The listing builds one solid part. Answer for the finished solid, in the listing's coordinates (mm). Coordinates: 2 decimals unless noted, no trailing zeros. Write each loop counter-clockwise with the first axis right and the second up, starting at its lowest first coordinate (ties: lowest second). Pieces come first, ordered by that corner, then holes. Notation, with made-up numbers: M 57.5,15 L 66.5,15 A17 ccw 66.5,32 Z; hole C -1,-38 d6. An arc over 180 degrees is marked long. Answer as CSV lines item,"result".
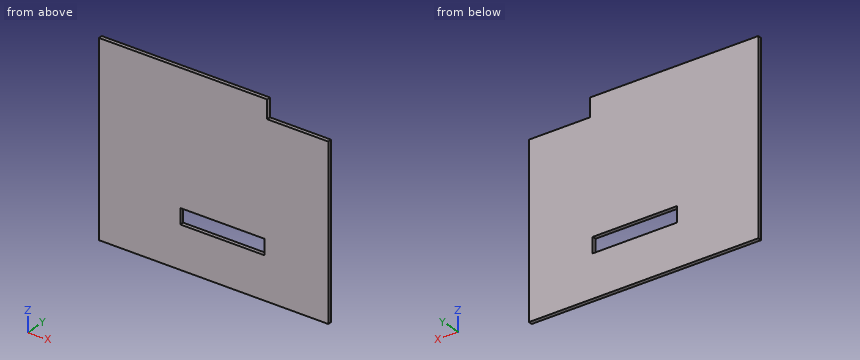
Autodesk Inventor part; units mm, degrees
ref_plane "YZ Plane" through (0, 0, 0) normal (1, 0, 0) x (0, 1, 0)
ref_plane "XZ Plane" through (0, 0, 0) normal (0, 1, 0) x (-1, 0, 0)
ref_plane "XY Plane" through (0, 0, 0) normal (0, 0, 1) x (1, 0, 0)
sketch "Esquisse1" plane through (0, 0, 0) normal (0, 1, 0) x (-1, 0, 0)
  line L0 (100.2268, 60.494) -> (-119.7732, 60.494)
  line L1 (-199.7732, 36.494) -> (-199.7732, -184.506)
  line L2 (-199.7732, -184.506) -> (100.2268, -184.506)
  line L3 (100.2268, -184.506) -> (100.2268, 60.494)
  line L4 (-119.7732, 60.494) -> (-119.7732, 36.494)
  line L5 (-119.7732, 36.494) -> (-199.7732, 36.494)
  point P0 (0, 0)
  dimension "d0" = 245
  dimension "d1" = 300
  dimension "d4" = 221
  dimension "d5" = 80
extrude "Extrusion1" add sketch "Esquisse1" along normal blind 5
sketch "Esquisse2" plane through (0, 5, 0) normal (0, 1, 0) x (1, 0, 0)
  line L0 (6.299, 109.506) -> (116.299, 109.506)
  line L1 (116.299, 109.506) -> (116.299, 129.506)
  line L2 (116.299, 129.506) -> (6.299, 129.506)
  line L3 (6.299, 129.506) -> (6.299, 109.506)
  line L4 (199.7732, 184.506) -> (-100.2268, 184.506)
  point P0 (0, 0)
  dimension "d6" = 20
  dimension "d7" = 110
  dimension "d8" = 55
extrude "Extrusion2" cut sketch "Esquisse2" against normal through all
properties part number "cote"
Q1. Find section C-C (y = 3.65). Give the vertices of the cut face in (x, z), and give its area (3 significant figures).
Output:
outline,"M -100.23,-184.51 L 199.77,-184.51 L 199.77,36.49 L 119.77,36.49 L 119.77,60.49 L -100.23,60.49 Z; hole M 6.3,-129.51 L 116.3,-129.51 L 116.3,-109.51 L 6.3,-109.51 Z"
area,"69,400 mm2"
Q2. Find section A-A (z = -116). Give the vertices of the cut face in (x, y), and give its area (3 significant figures).
Output:
outline,"M -100.23,0 L 6.3,0 L 6.3,5 L -100.23,5 Z; M 116.3,0 L 199.77,0 L 199.77,5 L 116.3,5 Z"
area,"950 mm2"
Q3. Flat-ended cylindrical pins translate along their axes: pin 1 Ø6 at (x, z) = (72.5, -113.5) entering from +Y; pin 2 Ø1.5 at (y, z) = (3, 46.5) entering from +X. Find the tip coordinate at first contact, or state that the pin passes through.
Output:
pin 1,"through"
pin 2,"x = 119.77"
Q4. Straight lines are drawn through the part: line 1 (X direction, y = 0.9, z = -128); line 2 (Z direction, x = 95.5, y = 4.5); line 3 (Z direction, x = 165, y = 1.6). For each, find the intervals that lie inside material, in ascending order.
Output:
line 1,"-100.23 to 6.3, 116.3 to 199.77"
line 2,"-184.51 to -129.51, -109.51 to 60.49"
line 3,"-184.51 to 36.49"
Q5. Find section B-B (x = 103.5). Give the vertices of the cut face in (y, z).
Output:
outline,"M 0,-184.51 L 5,-184.51 L 5,-129.51 L 0,-129.51 Z; M 0,-109.51 L 5,-109.51 L 5,60.49 L 0,60.49 Z"
Q6. Find section D-D (x = 144.5). Give the vertices of the cut face in (y, z).
Output:
outline,"M 0,-184.51 L 5,-184.51 L 5,36.49 L 0,36.49 Z"
